```python
from build123d import *

# Parameters (mm, degrees)
BOSS_EXTRUDE1_DEPTH = 20
FILLET2_R           = 5
FILLET3_R           = 5
FILLET4_R           = 5
FILLET5_R           = 3.5
CHAMFER1_SIZE       = 2
CHAMFER2_SIZE       = 0.75
CHAMFER3_SIZE       = 0.5


with BuildPart() as part:
    # Sketch1 → Boss-Extrude1 (new, symmetric)
    with BuildSketch(Plane(origin=(0, 0, 0), x_dir=(0, 0, -1), z_dir=(1, 0, 0))):
        Polygon((-69.940788655, 0), (-15, 0), (0, 0), (0, -40), (40, -40), (40, -26), (46, -26), (46, -46), (-6, -46), (-6, -3.95), (-13.226857143, -3.95), (-17.940788655, -3.95), (-17.940788655, -3.7), (-49.940788655, -3.7), (-49.940788655, -3.95), (-69.940788655, -3.95), align=None)
        Polygon((21, -72), (21, -46), (17, -46), (17, -76), (40.014855678, -76), (40.014855678, -66), (36.014855678, -66), (36.014855678, -72), align=None)
    extrude(amount=BOSS_EXTRUDE1_DEPTH, both=True)

    # Fillet2
    fillet2_edges = [part.edges().sort_by_distance(p)[0] for p in [
        (0, 0, 0),
    ]]
    fillet(fillet2_edges, radius=FILLET2_R)

    # Fillet3
    fillet3_edges = [part.edges().sort_by_distance(p)[0] for p in [
        (0, -40, 0),
        (0, -40, -40),
    ]]
    fillet(fillet3_edges, radius=FILLET3_R)

    # Fillet4
    fillet4_edges = [part.edges().sort_by_distance(p)[0] for p in [
        (0, -46, -46),
        (0, -46, 6),
    ]]
    fillet(fillet4_edges, radius=FILLET4_R)

    # Fillet5
    fillet5_edges = [part.edges().sort_by_distance(p)[0] for p in [
        (0, -72, -21),
        (0, -72, -36.014855678),
        (0, -76, -40.014855678),
        (0, -76, -17),
    ]]
    fillet(fillet5_edges, radius=FILLET5_R)

    # Chamfer1
    # the kernel refuses this chamfer: 2 mm, written as the material it takes off along each edge
    with BuildSketch(Plane(origin=(-25.143365976, -3.95, 69.940788655), x_dir=(0, 0.9996219169112968, 0.027495876610589075), z_dir=(1, 0, 0)), Plane(origin=(-25.143365976, 0, 69.940788655), x_dir=(0, 0.02749587661058631, -0.9996219169112968), z_dir=(1, 0, 0))) as chamfer1_piece_1:
        Polygon((CHAMFER1_SIZE * 0.999621916911, -CHAMFER1_SIZE * 0.0274958766106), (-CHAMFER1_SIZE * 0.0274958766106, -CHAMFER1_SIZE * 0.999621916911), (0, 0), align=None)
    extrude(amount=50.286731952, mode=Mode.SUBTRACT)

    # Chamfer2
    chamfer2_edges = [part.edges().sort_by_distance(p)[0] for p in [
        (0, -26, -40),
        (0, -26, -46),
    ]]
    chamfer(chamfer2_edges, length=CHAMFER2_SIZE)

    # Chamfer3
    chamfer3_edges = [part.edges().sort_by_distance(p)[0] for p in [
        (0, -66, -36.014855678),
        (0, -66, -40.014855678),
    ]]
    chamfer(chamfer3_edges, length=CHAMFER3_SIZE)


solid = part.part
```
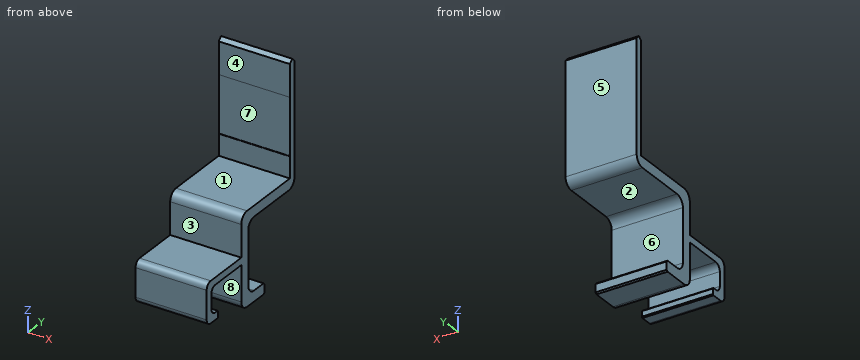
Input: part model. Units: mm. Frame: model coordinates. Face numbers are marked on the shaded views. A direction names the side the tool comes from. Give positions to 0.01 mm unless a question says otherwise; leave off trailing zeros. Order: outer loops, then holes, each group sorted by start corner. A loop starts at its lowest first (then second) coordinate and runs counter-clockwise, first axis right, second up. Notation, with made-up numbers: (-38.75, -37) - (-16.75, -37) arc R17 cw to (-16.75, -17) - close; hole circle Ø11 at (-5.75, 45). An arc over 180 degrees is marked (long way). Put each result on its own line as item: value.
Item 1: Draft query along Z for the marked faces 1, 2 and 3. Return one class per face: +Z half, -Z half, draft (parallel to the pull), parting line (faces both ways), or undercut.
Found:
face 1: +Z half
face 2: undercut
face 3: draft
Item 2: Section query A-A, the plane y = -16. Return loops of the section in (x, z).
Found:
outline: (-20, 0) - (20, 0) - (20, 6) - (-20, 6) - close
Item 3: Ray query, L1, parallel to Z at x = 12.5, y = -33; L2, parallel to Y at x = -12, z = 37; L3, parallel to Y at x = 18, z = -14. Return the intervals inside material, ascending. Write a range as from..to.
Found:
L1: z = -46..-40, 0..6
L2: y = -3.7..0
L3: y = -46..-40
Item 4: Section query B-B, the plane z = -2. Return loops of the section in (x, y), then the cut area to 3 significant figures.
Found:
outline: (-20, -46) - (20, -46) - (20, -39) - (-20, -39) - close
area: 280 mm^2
Item 5: Contact query for flat-ended pins moving along their axis: pin 1 (14.5 mm diameter, centred on x = -9, z = 61.5, fed in from -Y); pin 2 (1 mm diameter, centred on x = -12, y = -37.5, fed in from +Z); pin 3 (1 mm diameter, centred on x = -1, y = -67.5, fed in from +Z). Output: stop coordinate, or through.
Found:
pin 1: stops at y = -3.95
pin 2: stops at z = 6
pin 3: stops at z = -17
Item 6: Access query for the marked faces 4, 5, 6, 7 and 8. Directions: +Z, -Z, +X, -X, +Y, -Y. A direction counts if a zero-diameter tool reaches every point of the face in a straight line with its end or side. Return the directions, or none.
Found:
face 4: +Z, +X, -X, -Y
face 5: +Z, -Z, +X, -X, +Y
face 6: +X, -X, +Y
face 7: +X, -X, -Y
face 8: -Z, +X, -X
